For this review, take the finished solid that the model builds, in its own axes (mm). A direction names the side the tool comes from. Give positions to 0.01 mm unless a question says otherwise; leave off trailing zeros. Loops run counter-clockwise (first coordinate to the right, second up) from the corner with the lowest first, then second, coordinate; pieces in that order, holes last.
```python
from build123d import *

# Parameters (mm, degrees)
SKETCH1_W           = 63.5
SKETCH1_H           = 6.35
BOSS_EXTRUDE1_DEPTH = 12.7
SKETCH2_R           = 3.175
CUT_EXTRUDE1_DEPTH  = 26.162
FILLET1_R           = 6.35
SKETCH3_R           = 2.5796875
BOSS_EXTRUDE2_DEPTH = 12.7
FILLET2_R           = 12.7


with BuildPart() as part:
    # Sketch1 → Boss-Extrude1 (new body)
    with BuildSketch(Plane.XY):
        with Locations((31.75, -3.175)):
            Rectangle(SKETCH1_W, SKETCH1_H)
    extrude(amount=BOSS_EXTRUDE1_DEPTH)

    # Sketch2 → Cut-Extrude1 (cut)
    with BuildSketch(Plane(origin=(0, 0, 0), x_dir=(1, 0, 0), z_dir=(0, 1, 0))):
        with Locations(Location((8.255, -6.35, 0), (0, 0, 180))):
            Circle(SKETCH2_R)
        with Locations(Location((55.245, -6.35, 0), (0, 0, 180))):
            Circle(SKETCH2_R)
    extrude(amount=-CUT_EXTRUDE1_DEPTH, mode=Mode.SUBTRACT)

    # Fillet1
    fillet1_edges = [part.edges().sort_by_distance(p)[0] for p in [
        (63.5, -3.175, 12.7),
        (63.5, -3.175, 0),
        (0, -3.175, 0),
        (0, -3.175, 12.7),
    ]]
    fillet(fillet1_edges, radius=FILLET1_R - 0.0001)  # a hair under: the kernel refuses the full size

    # Sketch3 → Boss-Extrude2 (add)
    with BuildSketch(Plane.XY.offset(12.7)):
        with BuildLine():
            Line((25.4, -6.35), (38.1, -6.35))
            Line((38.1, -6.35), (38.1, -12.7))
            ThreePointArc((38.1, -12.7), (31.75, -19.05), (25.4, -12.7))
            Line((25.4, -12.7), (25.4, -6.35))
        make_face()
        with Locations((31.75, -12.7)):
            Circle(SKETCH3_R, mode=Mode.SUBTRACT)
    extrude(amount=-BOSS_EXTRUDE2_DEPTH)

    # Fillet2
    fillet2_edges = [part.edges().sort_by_distance(p)[0] for p in [
        (38.1, -6.35, 6.35),
        (25.4, -6.35, 6.35),
    ]]
    fillet(fillet2_edges, radius=FILLET2_R)


solid = part.part
```
Item 1: Take a section at B-B on x = 9.5. Give the boundary of the cut face in (y, z).
Answer:
outline: (-6.35, 0) - (0, 0) - (0, 3.43) - (-6.35, 3.43) - close; (-6.35, 9.27) - (0, 9.27) - (0, 12.7) - (-6.35, 12.7) - close
Item 2: Tool access review of faces 4 (the flat face through (58, -6.35, 9)), 5 (the cylindrical face through (6.55, -3.13, 9.03)), 6 (the flat face through (5, -6.35, 5)): name each direction out of +Z, -Z, +X, -X, +Y, -Y from which nothing blocks a thin tool from reaching the whole face with its end or side.
Answer:
face 4: +Z, -Z, +X, -Y
face 5: +Y, -Y
face 6: +Z, -Z, -X, -Y
Item 3: Take a section at A-A on x = 31.75. Give the boundary of the cut face in (y, z).
Answer:
outline: (-19.05, 0) - (-15.28, 0) - (-15.28, 12.7) - (-19.05, 12.7) - close; (-10.12, 0) - (0, 0) - (0, 12.7) - (-10.12, 12.7) - close
Item 4: Clearance check with flat-ended pins moving along their axes: pin 1 Ø4 at (x, z) = (57, 7) entering from -Y; pin 2 Ø3 at (x, z) = (45.5, 3) entering from -Y. State where each tip first meets the part, or that it passes through.
Answer:
pin 1: stops at y = -6.35
pin 2: stops at y = -7.71
Item 5: Take a section at C-C on y = -17.25. Give the boundary of the cut face in (x, z), and give its area (3 significant figures).
Answer:
outline: (27.32, 0) - (36.18, 0) - (36.18, 12.7) - (27.32, 12.7) - close
area: 113 mm2
Item 6: For L1, parallel to Y at x = 31.75, z = 3.25; L2, parallel to X at y = -2.5, z = 7.5; L3, parallel to X at y = -0.75, z = 4, list the stretches that pass through material, from the lowest coordinate up.
Answer:
L1: y = -19.05 to -15.28, -10.12 to 0
L2: x = 0.1 to 5.3, 11.21 to 52.29, 58.2 to 63.4
L3: x = 0.45 to 6.12, 10.39 to 53.11, 57.38 to 63.05
Item 7: The part is to be moulded in two halves that separate along Z. For faces 1 (the cylindrical face through (31.86, -19.05, 6.44)), 2 (the cylindrical face through (53.54, -3.13, 9.03)), 3 (the cylindrical face through (1.81, -3.13, 10.79)), say which applies: released by +Z, released by -Z, zero draft, split by the parting line, or undercut.
Answer:
face 1: zero draft
face 2: undercut
face 3: released by +Z
